```python
from build123d import *

# Parameters (mm, degrees)
SZKIC1_R                    = 4
SZKIC1_R_2                  = 2
DODANIE_WYCI_GNI_CIE1_DEPTH = 6
SZKIC2_W                    = 6
SZKIC2_H                    = 8
DODANIE_WYCI_GNI_CIE2_DEPTH = 10


with BuildPart() as part:
    # Szkic1 → Dodanie-wyciągnięcie1 (new body)
    # profile 1 of 2: a face of its own
    with BuildSketch(Plane(origin=(0, 0, 0), x_dir=(0, 0, -1), z_dir=(1, 0, 0))):
        with BuildLine():
            Line((46, 4), (0, 4))
            ThreePointArc((0, 4), (2.828427125, 2.828427125), (4, 0))
            ThreePointArc((4, 0), (2.828427125, -2.828427125), (0, -4))
            Line((0, -4), (46, -4))
            Line((46, -4), (46, 4))
        make_face()
    # profile 2 of 2: a face of its own
    with BuildSketch(Plane(origin=(0, 0, 0), x_dir=(0, 0, -1), z_dir=(1, 0, 0))):
        Circle(SZKIC1_R)
        Circle(SZKIC1_R_2, mode=Mode.SUBTRACT)
    extrude(amount=DODANIE_WYCI_GNI_CIE1_DEPTH)

    # Szkic2 → Dodanie-wyciągnięcie2 (add)
    with BuildSketch(Plane(origin=(6, 0, 0), x_dir=(0, 0, -1), z_dir=(1, 0, 0))):
        with Locations((43, 0)):
            Rectangle(SZKIC2_W, SZKIC2_H)
    extrude(amount=DODANIE_WYCI_GNI_CIE2_DEPTH)


solid = part.part
```
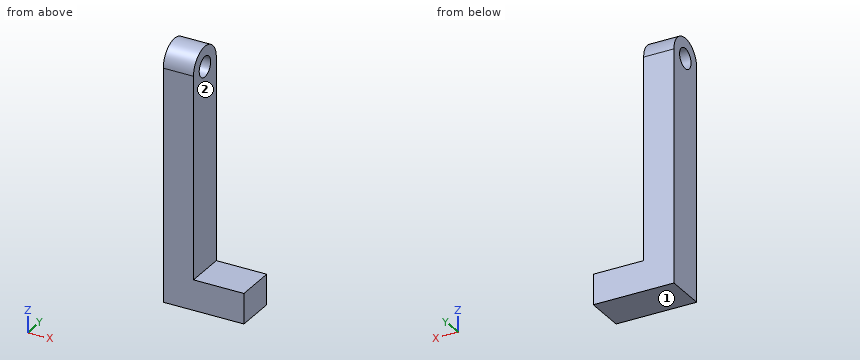
Geometry check sheet. Reference: the model listing, model coordinates, mm. Face numbers are marked on the shaded views. A direction names the side the tool comes from. Give positions to 0.01 mm unless a question says otherwise; leave off trailing zeros. Order: outer loops, then holes, each group sorted by start corner. A loop starts at its lowest first (then second) coordinate and runs counter-clockwise, first axis right, second up. Notation, with made-up numbers: (35.25, -33) -> (74.25, -33) arc R21 cw to (74.25, -15) -> close; hole circle Ø6 at (19.25, 3.25). An arc over 180 degrees is marked (long way). Write each question's results on one line, items separated by ' | '. Start each with the question number.
(1) Scan lines: line 1 (X direction, y = 0.5, z = -16.5); line 2 (Z direction, x = 15.25, y = 1.75); line 3 (Y direction, x = 3.35, z = 0). Record each from-to range of solid material in increasing order.
(2) Access from +Z, -Z, +X, -X, +Y, -Y to the whole of each face (thin tool, end or side, straight path). Record for the marked faces 1 and 2.
(3) Sectioned sample at A-A (y = 0). Enter the section's corners in (x, z), plus the area to 3 significant figures.
(4) Sectioned sample at D-D (y = 3). Enter the section's corners in (x, z), plus the area to 3 significant figures.
(5) Gauge pin test, flat ends, axial feed: P1, Ø4, axis at y = -1.5, z = -22, coming from the +X side; P2, Ø2.5, axis at x = 11, y = 1, coming from the +Z side. Record the tip position at first contact, or that the pin passes through.
(6) Sectioned sample at C-C (z = -23). Enter the section's corners in (x, y), plus the area to 3 significant figures.
(7) Sectioned sample at B-B (x = 5). Enter the section's corners in (y, z).
Answer below:
1) line 1: 0 to 6 | line 2: -46 to -40 | line 3: -4 to -2, 2 to 4
2) face 1: -Z, +X, -X, +Y, -Y | face 2: +Z, +X, +Y, -Y
3) outline: (0, -46) -> (16, -46) -> (16, -40) -> (6, -40) -> (6, -2) -> (0, -2) -> close; (0, 2) -> (6, 2) -> (6, 4) -> (0, 4) -> close | area: 336 mm2
4) outline: (0, -46) -> (16, -46) -> (16, -40) -> (6, -40) -> (6, 2.65) -> (0, 2.65) -> close | area: 352 mm2
5) P1: x = 6 | P2: z = -40
6) outline: (0, -4) -> (6, -4) -> (6, 4) -> (0, 4) -> close | area: 48.0 mm2
7) outline: (-4, -46) -> (4, -46) -> (4, 0) arc R4 ccw to (-4, 0) -> close; hole circle Ø4 at (0, 0)
